Autodesk Inventor part; units mm, degrees
ref_plane "YZ Plane" through (0, 0, 0) normal (1, 0, 0) x (0, 1, 0)
ref_plane "XZ Plane" through (0, 0, 0) normal (0, 1, 0) x (-1, 0, 0)
ref_plane "XY Plane" through (0, 0, 0) normal (0, 0, 1) x (1, 0, 0)
sketch "Sketch1" plane through (0, 0, 0) normal (1, 0, 0) x (0, 1, 0)
  line L0 (0, 0) -> (3, 0)
  line L1 (3, 0) -> (3, -19) construction
  line L2 (3, -19) -> (0, -19)
  line L3 (0, -19) -> (0, 0)
  line L4 (3, 0) -> (3, 3) construction
  line L5 (3, 3) -> (23.0125, 3) construction
  line L6 (33, 3) -> (33, -22) construction
  line L7 (33, -22) -> (23.0125, -22) construction
  line L8 (3, -22) -> (3, -19)
  line L9 (33, -9.5) -> (40.75, -9.5) construction
  line L10 (40.75, -9.5) -> (40.75, -17.25) construction
  line L11 (40.75, -17.25) -> (33, -17.25) construction
  line L12 (33, -17.25) -> (33, -9.5) construction
  circle A0 centre (40.75, -17.25) radius 1.5
  line L13 (40.75, -17.25) -> (25.25, -17.25) construction
  line L14 (25.25, -17.25) -> (25.25, -1.75) construction
  line L15 (25.25, -1.75) -> (40.75, -1.75) construction
  line L16 (40.75, -1.75) -> (40.75, -17.25) construction
  circle A1 centre (25.25, -17.25) radius 1.5
  circle A2 centre (25.25, -1.75) radius 1.5
  circle A3 centre (40.75, -1.75) radius 1.5
  arc A4 (23.0125, -22) -> (23.0125, 3) centre (33, -9.5) ccw
  line L17 (23.0125, 3) -> (33, 3) construction
  line L18 (23.0125, -22) -> (3, -22) construction
  arc A5 (3, 3) -> (23.0125, 3) centre (13.0063, 17.9624) ccw
  arc A6 (23.0125, -22) -> (3, -22) centre (13.0063, -36.9624) ccw
  line L19 (3, 0) -> (3, 3)
  line L20 (3, -19) -> (3, 0) construction
  arc A7 (23.0125, 3) -> (23.0125, -22) centre (33, -9.5) ccw construction
  point P0 (23.0125, -22)
  point P1 (23.0125, 3)
  dimension "d0" = 3
  dimension "d1" = 19
  dimension "d2" = 3
  dimension "d3" = 30
  dimension "d4" = 25
  dimension "d5" = 7.75
  dimension "d6" = 7.75
  dimension "d7" = 3
  dimension "d8" = 15.5
  dimension "d9" = 15.5
  dimension "d10" = 3
  dimension "d11" = 3
  dimension "d12" = 3
  dimension "d13" = 32
  dimension "d16" = 18
  dimension "d17" = 18
extrude "Extrusion1" add sketch "Sketch1" along normal blind 3
properties part number "soporteEncoder" material "PMMA Plastic"
The model under review builds one solid part; all positions refer to its coordinate system, in mm. A direction names the side the tool comes from. Coordinates: 2 decimals unless noted, no trailing zeros. Loops run counter-clockwise (first coordinate to the right, second up) from the corner with the lowest first, then second, coordinate; pieces in that order, holes last. Notation, with made-up numbers: (18.25, 21) -> (41.25, 21) arc R34 cw to (41.25, 51) -> close; hole circle Ø8 at (-33.75, 29). An arc over 180 degrees is marked (long way). Use a Markdown table: item, result. Add a question column.
1. Add section C-C on z = -17.25. Write out the cut boundary in (x, y).
2. Draft analysis for pull direction Z (two halves, no side actions). For faces 4 (the face through (1.48, 23.75, -1.82)), 5 (the face through (1, 1, 0)), 6 (the face through (1.479, 48.992, -8.997)), 7 (the face through (1, 3, -21)), state which applies: pulls with the +Z half, pulls with the -Z half, needs draft (parallel to the pull), parting line crosses it, or undercut.
3. Machinability: for faces 1 (the face through (1, 3, 1)), 2 (the face through (1, 2, -19)), 3 (the face through (1, 0, -10)), which of the approach directions +Z, -Z, +X, -X, +Y, -Y give a long, thin tool a straight path to every point of the face, cutting with its end or side? Answer none if there is none.
4. Add section B-B on y = 25.25. Write out the cut boundary in (x, z).
5. Add section A-A on x = 1.15. Write out the cut boundary in (y, z), plus the area to 3 significant figures.
6. Add section D-D on y = 9. Write out the cut boundary in (x, z).
7. To check wall thickness, follow line 1 (Z direction, x = 1.6, y = 40); line 2 (Z direction, x = 2.4, y = 24); line 3 (Y direction, x = 1.7, z = -2.5). State the ranges of each line that lie inside material, in increasing order.
8. Clearance check with flat-ended pins moving along their axes: pin 1 Ø0.9 at (x, y) = (1.5, 2) entering from -Z; pin 2 Ø1.8 at (y, z) = (40.75, -1.75) entering from -X; pin 3 Ø1.5 at (x, y) = (2, 2) entering from +Z; pin 4 Ø1.5 at (x, z) = (1.5, 2) entering from -Y. State where each tip first meets the part, or that it passes through.
Returned:
| question | item | result |
|---|---|---|
| 1 | outline | (0, 0) -> (3, 0) -> (3, 23.75) -> (0, 23.75) -> close; (0, 26.75) -> (3, 26.75) -> (3, 39.25) -> (0, 39.25) -> close; (0, 42.25) -> (3, 42.25) -> (3, 47) -> (0, 47) -> close |
| 2 | face 4 | undercut |
| 2 | face 5 | pulls with the +Z half |
| 2 | face 6 | parting line crosses it |
| 2 | face 7 | needs draft |
| 3 | face 1 | +Z, +X, -X, -Y |
| 3 | face 2 | -Z, +X, -X, -Y |
| 3 | face 3 | +Z, -Z, +X, -X, -Y |
| 4 | outline | (0, -23.5) -> (3, -23.5) -> (3, -18.75) -> (0, -18.75) -> close; (0, -15.75) -> (3, -15.75) -> (3, -3.25) -> (0, -3.25) -> close; (0, -0.25) -> (3, -0.25) -> (3, 4.5) -> (0, 4.5) -> close |
| 5 | outline | (0, -19) -> (3, -19) -> (3, -22) arc R18 cw to (23.01, -22) arc R16 ccw (long way) to (23.01, 3) arc R18 cw to (3, 3) -> (3, 0) -> (0, 0) -> close; hole circle Ø3 at (25.25, -17.25); hole circle Ø3 at (25.25, -1.75); hole circle Ø3 at (40.75, -17.25); hole circle Ø3 at (40.75, -1.75) |
| 5 | area | 1,150 mm² |
| 6 | outline | (0, -19.41) -> (3, -19.41) -> (3, 0.41) -> (0, 0.41) -> close |
| 7 | line 1 | z = -23.89 to -18.55, -15.95 to -3.05, -0.45 to 4.89 |
| 7 | line 2 | z = -22.73 to -18.08, -16.42 to -2.58, -0.92 to 3.73 |
| 7 | line 3 | y = 0 to 23.95, 26.55 to 39.45, 42.05 to 47.39 |
| 8 | pin 1 | stops at z = -19 |
| 8 | pin 2 | passes through |
| 8 | pin 3 | stops at z = 0 |
| 8 | pin 4 | stops at y = 3 |
